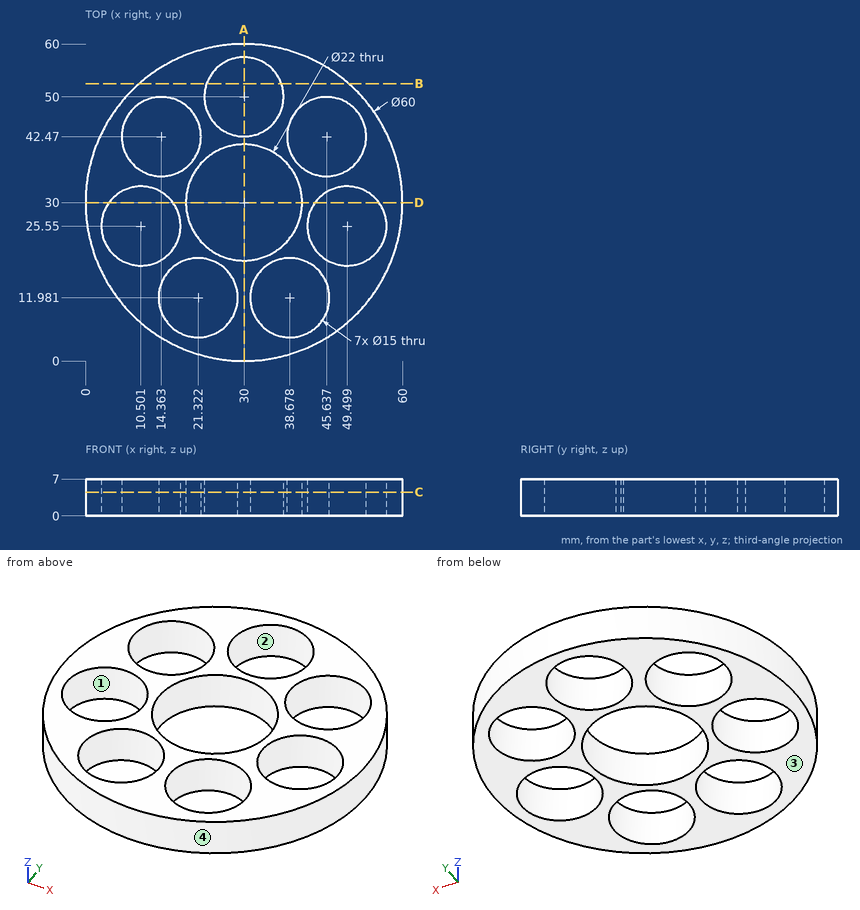
Design review of the part shown in the three views and the two pictorial views. Dimensions are in mm from the part's minimum x, y and z. Give positions to 0.01 mm unless a question says otherwise; leave off trailing zeros. Order: outer loops, then holes, each group sorted by start corner. A loop starts at its lowest first (then second) coordinate and runs counter-clockwise, first axis right, second up. Notation, with made-up numbers: M -8.5,44 L 41.5,44 A12 ccw 41.5,61 Z; hole C 48,71.5 d9. An arc over 180 degrees is marked long. Answer in a Markdown table with one row per item. Add a question column.
(1) Consider section A-A on x = 30. State the section outline as (y, z) points.
(2) Consider section C-C on z = 4.5. Give the number of separate pieces and of enclosed holes in the cut face, and give its area (3 significant figures).
(3) For pin 1 (4 mm diameter, centred on x = 36.5, z = 1, fed in from -Y), flat-tipped, find the tip position at first contact; note if it passes through.
(4) Consider section B-B on y = 52.5. State the section outline as (x, z) points.
(5) Mouldability with a two-part tool opening along X and no side actions: class the marked faces 1, 2, 3 and 4 as +X half, -X half, draft (parallel to the pull), parting line (faces both ways), or undercut.
(6) Consider section D-D on y = 30. State the section outline as (x, z) points (1 decimal).
(7) Wall thickness on probe 1 along X at (y, z) = (12.5, 2.5) (1 decimal); probe 2 along X at (y, z) = (48, 2.25) (1 decimal); probe 3 along Y at (x, z) = (29, 3.5) (1 decimal): over which ranges is each line inside the solid? List them lowest first. Write a range as [from, to].
Evaluation:
| question | item | result |
|---|---|---|
| 1 | outline | M 0,0 L 19,0 L 19,7 L 0,7 Z; M 41,0 L 42.5,0 L 42.5,7 L 41,7 Z; M 57.5,0 L 60,0 L 60,7 L 57.5,7 Z |
| 2 | separate pieces | 1 |
| 2 | enclosed holes | 8 |
| 2 | area | 1,210 mm^2 |
| 3 | pin 1 | stops at y = 0.34 |
| 4 | outline | M 10.16,0 L 22.93,0 L 22.93,7 L 10.16,7 Z; M 37.07,0 L 49.84,0 L 49.84,7 L 37.07,7 Z |
| 5 | face 1 | undercut |
| 5 | face 2 | undercut |
| 5 | face 3 | draft |
| 5 | face 4 | parting line |
| 6 | outline | M 0,0 L 4.5,0 L 4.5,7 L 0,7 Z; M 16.5,0 L 19,0 L 19,7 L 16.5,7 Z; M 41,0 L 43.5,0 L 43.5,7 L 41,7 Z; M 55.5,0 L 60,0 L 60,7 L 55.5,7 Z |
| 7 | probe 1 | x = [5.6, 13.8], [28.8, 31.2], [46.2, 54.4] |
| 7 | probe 2 | x = [6, 9.3], [19.4, 22.8], [37.2, 40.6], [50.7, 54] |
| 7 | probe 3 | y = [0, 19], [41, 42.6], [57.4, 60] |
